from build123d import *

# Parameters (mm, degrees)
F0_R          = 2.5
F1_DEPTH      = 10
F1_DEPTH_BACK = 6
F2_SIZE       = 1
F0_W          = 6
F0_H          = 6
F3_DEPTH      = 6
F4_SIZE       = 0.49999


# Not quite as in the source:
# - a fillet or chamfer is up to 0.001 mm smaller than in the source, because OpenCascade refuses the exact size


with BuildPart() as f1:
    # F0 (on Front) → F1 (new body, two sides)
    with BuildSketch(Plane.XZ) as f1_sk:
        Circle(F0_R)
    extrude(amount=-F1_DEPTH)
    extrude(f1_sk.sketch, amount=F1_DEPTH_BACK)

    # F2
    f2_edges = [f1.edges().sort_by_distance(p)[0] for p in [
        (-2.5, 10, 0),
    ]]
    chamfer(f2_edges, length=F2_SIZE)

    # F0 (on Front) → F3 (join)
    with BuildSketch(Plane.XZ):
        Rectangle(F0_W, F0_H)
        Circle(F0_R, mode=Mode.SUBTRACT)
    extrude(amount=F3_DEPTH)

    # F4 (size 0.5 in the source; OpenCascade refuses exactly that, so slightly less here)
    f4_edges = [f1.edges().sort_by_distance(p)[0] for p in [
        (3, -6, 0),
        (0, -6, 3),
        (-3, -6, 0),
        (0, -6, -3),
        (3, 0, 0),
        (-3, 0, 0),
        (0, 0, 3),
        (0, 0, -3),
    ]]
    chamfer(f4_edges, length=F4_SIZE)


solid = f1.part
Geometry check sheet. Reference: the model listing, model coordinates, mm. A direction names the side the tool comes from. Give positions to 0.01 mm unless a question says otherwise; leave off trailing zeros. Loops run counter-clockwise (first coordinate to the right, second up) from the corner with the lowest first, then second, coordinate; pieces in that order, holes last. Notation, with made-up numbers: M 48,74 L 88,74 A17 cw 88,105 Z; hole C 80,-21 d4. An arc over 180 degrees is marked long. Answer as a JSON object with one key per item and string values. Group by question number.
Item 1: Access from +Z, -Z, +X, -X, +Y, -Y to the whole of each face (thin tool, end or side, straight path). Record for faces 1 (the cylindrical face through (-0.54, 4.44, -2.44)), 2 (the flat face through (-3, -3, 0)).
Item 2: Sectioned sample at C-C on y = 2. Record the boundary of the cut face in (x, z).
Item 3: Gauge pin test, flat ends, axial feed: pin 1 (1 mm diameter, centred on x = -1.5, z = 1, fed in from +Y); pin 2 (1.5 mm diameter, centred on x = 1.5, y = 6.5, fed in from +Z); pin 3 (1 mm diameter, centred on x = -1, z = -2.5, fed in from +Y); pin 4 (2 mm diameter, centred on x = 2, y = 3, fed in from +Z). Record the tip position at first contact, or that the pin passes through.
Item 4: Material ranges on L1, parallel to Z at x = 2, y = 1; L2, parallel to X at y = 6, z = -1, recorded low to high.
Findings below:
{
 "1": {"face 1": "+Y", "face 2": "+Z, -Z, -X, +Y, -Y"},
 "2": {"outline": "C 0,0 d5"},
 "3": {"pin 1": "y = 10", "pin 2": "z = 2.38", "pin 3": "y = 9.31", "pin 4": "z = 2.29"},
 "4": {"L1": "-1.5 to 1.5", "L2": "-2.29 to 2.29"}
}
